Autodesk Inventor part; units mm, degrees
ref_plane "YZ Plane" through (0, 0, 0) normal (1, 0, 0) x (0, 1, 0)
ref_plane "XZ Plane" through (0, 0, 0) normal (0, 1, 0) x (-1, 0, 0)
ref_plane "XY Plane" through (0, 0, 0) normal (0, 0, 1) x (1, 0, 0)
sketch "Sketch1" plane through (0, 0, 0) normal (0, 1, 0) x (-1, 0, 0)
  circle A0 centre (0, 0) radius 22.86
  line L0 (14.5416, -26.67) -> (-16.51, -26.67)
  line L1 (-20.32, -15.24) -> (-20.32, -55.88)
  line L2 (-13.6865, -63.5) -> (16.51, -63.5)
  line L3 (20.32, -55.88) -> (20.32, -15.24)
  line L4 (16.51, -67.31) -> (-16.51, -67.31)
  line L5 (-20.32, -59.69) -> (-20.32, -100.33)
  line L6 (-16.51, -104.14) -> (13.9515, -104.14)
  line L7 (20.32, -100.33) -> (20.32, -59.69)
  line L8 (13.9515, -107.95) -> (-16.51, -107.95)
  line L9 (-20.32, -104.14) -> (-20.32, -144.78)
  line L10 (20.32, -144.78) -> (20.32, -104.14)
  line L11 (20.32, -15.24) -> (20.32, -10.4727)
  circle A1 centre (0, -163.83) radius 6.35
  line L12 (-20.32, -15.24) -> (-20.32, -10.4727)
  line L13 (20.32, -55.88) -> (20.32, -59.69)
  line L14 (20.32, -100.33) -> (20.32, -104.14)
  line L15 (-20.32, -55.88) -> (-20.32, -59.69)
  line L16 (-20.32, -100.33) -> (-20.32, -104.14)
  line L17 (20.32, -144.78) -> (20.32, -148.59)
  line L18 (-20.32, -144.78) -> (-20.32, -148.59)
  line L19 (20.32, -148.59) -> (8.7779, -160.1321)
  line L20 (-20.32, -148.59) -> (-8.7779, -160.1321)
  line L21 (16.51, -30.1719) -> (16.51, -63.5)
  line L22 (-16.51, -26.67) -> (-16.51, -60.9418)
  line L23 (16.51, -67.31) -> (16.51, -101.2863)
  line L24 (-16.51, -67.31) -> (-16.51, -104.14)
  line L25 (16.51, -110.8037) -> (16.51, -144.78)
  line L26 (-16.51, -141.9263) -> (-16.51, -107.95)
  arc A2 (-8.7779, -160.1321) -> (8.7779, -160.1321) centre (0, -163.83) ccw
  line L27 (14.5416, -26.67) -> (-16.51, -60.9418)
  line L28 (16.9388, -26.8614) -> (16.51, -27.3347)
  line L29 (17.3651, -29.2282) -> (-13.6865, -63.5)
  line L30 (-13.9515, -67.31) -> (16.51, -101.2863)
  line L31 (-16.51, -70.1637) -> (13.9515, -104.14)
  line L32 (13.9515, -107.95) -> (-16.51, -141.9263)
  line L33 (16.51, -110.8037) -> (-13.9515, -144.78)
  line L34 (-19.0685, -144.78) -> (-16.51, -144.78)
  line L35 (-13.9515, -144.78) -> (16.51, -144.78)
  dimension "d0" = 45.72
  dimension "d2" = 26.67
  dimension "d3" = 36.83
  dimension "d5" = 20.32
  dimension "d6" = 3.81
  dimension "d7" = 40.64
  dimension "d8" = 3.81
  dimension "d10" = 12.7
  dimension "d11" = 3.81
  dimension "d12" = 3.81
  dimension "d13" = 135
  dimension "d14" = 3.81
  dimension "d15" = 3.81
  dimension "d16" = 3.81
  dimension "d17" = 36.83
  dimension "d19" = 94.2927
  dimension "d20" = 62.8618
  dimension "d21" = 123.0295
  dimension "d22" = 94.2927
  dimension "d23" = 91.5986
  dimension "d24" = 62.8618
  dimension "d25" = 3.81
  dimension "d26" = 36.83
  dimension "d27" = 65.5559
  dimension "d28" = 60.1677
  dimension "d29" = 19.05
  dimension "d32" = 1.905
  dimension "d37" = 42.178
  dimension "d38" = 138.122
  dimension "d39" = 138.122
  dimension "d40" = 118.11
  dimension "d41" = 36.83
  dimension "d42" = 0
  dimension "d43" = 3.81
  dimension "d44" = 3.81
  dimension "d45" = 86.2593
  dimension "d46" = 55.3203
  dimension "d47" = 3.3812
  dimension "d48" = 11.5421
  dimension "d49" = 36.83
  dimension "d50" = 119.4374
  dimension "d51" = 119.4374
  dimension "d52" = 20.32
extrude "Extrusion1" add sketch "Sketch1" along normal blind 22.225
sketch "Sketch2" plane through (0, 22.225, 0) normal (0, 1, 0) x (1, 0, 0)
  circle A0 centre (0, 0) radius 18.415
  dimension "d55" = 36.83
extrude "Extrusion2" cut sketch "Sketch2" against normal blind 17.907
sketch "Sketch3" plane through (0, 4.318, 0) normal (0, 1, 0) x (1, 0, 0)
  circle A0 centre (0, -6.985) radius 6.096
  line L0 (0, 0) -> (0, -18.9723)
  arc A1 (-20.32, 10.4727) -> (20.32, 10.4727) centre (0, 0) ccw
  line L1 (-15.494, 0) -> (15.494, 0)
  circle A2 centre (-15.494, 0) radius 1.9939
  circle A3 centre (15.494, 0) radius 1.9939
  point P0 (0, -22.86)
  dimension "d58" = 6.985
  dimension "d59" = 12.192
  dimension "d61" = 3.9878
  dimension "d62" = 30.988
  dimension "d63" = 15.494
  dimension "d65" = 18.9722
extrude "Extrusion3" cut sketch "Sketch3" against normal blind 36.322
properties part number "leg 3.0"
For this review, take the finished solid that the model builds, in its own axes (mm). A direction names the side the tool comes from. Coordinates: 2 decimals unless noted, no trailing zeros. Loops run counter-clockwise (first coordinate to the right, second up) from the corner with the lowest first, then second, coordinate; pieces in that order, holes last.
1. For faces 1 (the flat face through (20.32, 11, -80)), 2 (the flat face through (-1, 11, -144.78)), list the 3-axis set-ups (+Z, -Z, +X, -X, +Y, -Y) from which the entire face can be reached by the end or side of a thin tool; tool diameter is ignored.
2. Mouldability with a two-part tool opening along X and no side actions: class faces 3 (the flat face through (14.63, 10.96, -154.28)), 4 (the flat face through (1, 11, -107.95)), 5 (the flat face through (-20.32, 11, -80)), 6 (the flat face through (16.51, 11, -125)) as +X half, -X half, draft (parallel to the pull), parting line (faces both ways), or undercut.
3. For line 1 (X direction, y = 1.3, z = 0); line 2 (X direction, y = 3.75, z = -60); line 3 (Z direction, x = -15, y = 14.75), list the stretches that pass through material, from the lowest coordinate up.
4. Add section B-B, the plane y = 7.75. Count the separate pieces of the cut face and the enclosed holes in it, then the cut area to 3 significant figures.
5. Add section C-C, the plane z = -81. Give the boundary of the cut face in (x, y) (3 decimals), then the cut area to 3 significant figures.
6. Add section A-A, the plane z = -163.83. Give the boundary of the cut face in (x, y) (3 decimals), then the cut area to 3 significant figures.
7. Insertion check: P1, Ø12, axis at y = 17, z = -31, coming from the -X side; P2, Ø12, axis at y = 3.5, z = -144, coming from the +X side; P3, Ø19.5, axis at x = 0, z = 6.985, coming from the +Y side. Each pin has a flat end and moves straight along its axis. Give the tip position at first contact, or say it passes through.
Result:
1. face 1: -Z, +X, +Y, -Y
1. face 2: +Y, -Y
2. face 3: +X half
2. face 4: undercut
2. face 5: -X half
2. face 6: undercut
3. line 1: x = -22.86 to -17.49, -13.5 to 13.5, 17.49 to 22.86
3. line 2: x = -20.32 to -16.51, 10.52 to 15.66, 16.51 to 20.32
3. line 3: z = -153.91 to -144.78, -112.49 to -99.6, -67.31 to -63.5, -31.84 to -10.68, 10.68 to 17.25
4. separate pieces: 1
4. enclosed holes: 8
4. area: 3,150 mm2
5. outline: (-20.32, 0) - (-16.51, 0) - (-16.51, 22.225) - (-20.32, 22.225) - close; (1.678, 0) - (6.795, 0) - (6.795, 22.225) - (1.678, 22.225) - close; (16.51, 0) - (20.32, 0) - (20.32, 22.225) - (16.51, 22.225) - close
5. area: 283 mm2
6. outline: (-9.525, 0) - (-6.35, 0) - (-6.35, 22.225) - (-9.525, 22.225) - close; (6.35, 0) - (9.525, 0) - (9.525, 22.225) - (6.35, 22.225) - close
6. area: 141 mm2
7. P1: stops at x = -20.32
7. P2: stops at x = 20.32
7. P3: stops at y = 4.32
